Geometry check sheet. Reference: drawing and pictorial views, mm from the part's lowest x, y, z. A direction names the side the tool comes from. Coordinates: 2 decimals unless noted, no trailing zeros. Loops run counter-clockwise (first coordinate to the right, second up) from the corner with the lowest first, then second, coordinate; pieces in that order, holes last. Notation, with made-up numbers: M 62,-15.75 L 88,-15.75 A18 cw 88,-1.75 Z; hole C -14.75,61 d4. An arc over 180 degrees is marked long. Write item = value, one per line. Start each with the question number.
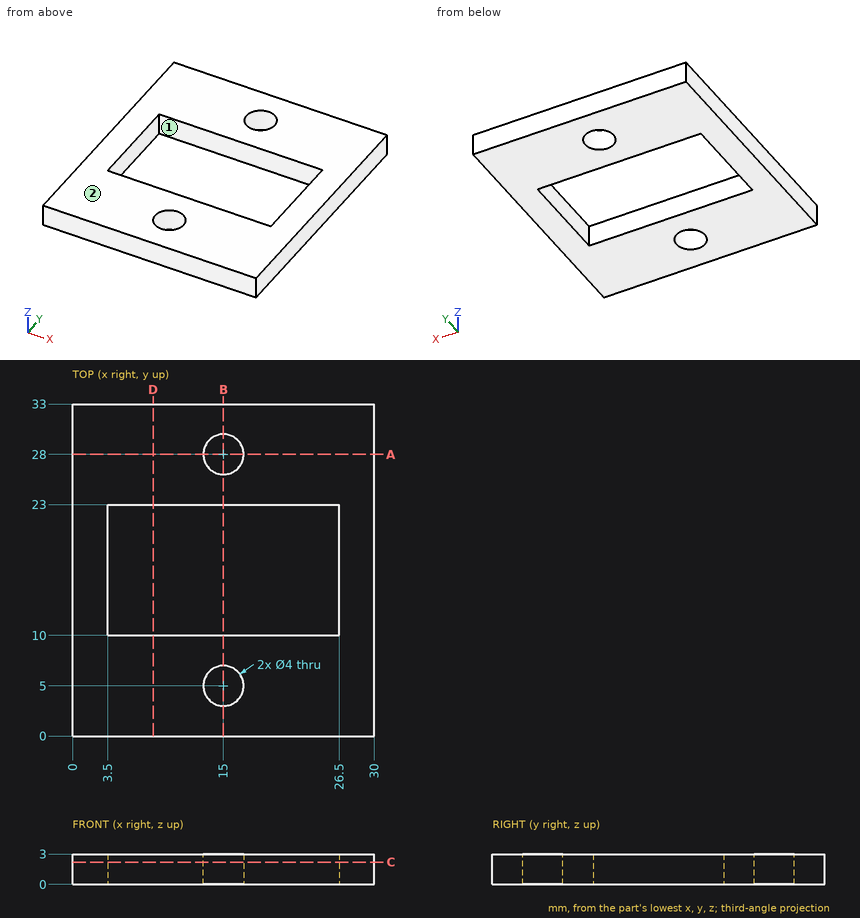
Q1. Scan lines: L1, parallel to Y at x = 15, z = 1.55; L2, parallel to Y at x = 5.75, z = 1.7; L3, parallel to X at y = 11, z = 0.5. Record each from-to range of solid material in increasing order. Write a range as [from, to].
Q2. Gauge pin test, flat end, axial feed: pin 1 (4.5 mm diameter, centred on x = 15, y = 28, fed in from +Z). Record the tip position at first contact, or that the pin passes through.
Q3. Sectioned sample at B-B on x = 15. Record the cut outline in (y, z), plus the area to 3 significant figures.
Q4. Sectioned sample at D-D on x = 8. Record the cut outline in (y, z).
Q5. Set-up check for the marked faces 1 and 2: record each of +Z, -Z, +X, -X, +Y, -Y from which the full face is reachable in a straight line by a thin tool's end or side.
Q6. Sectioned sample at A-A on y = 28. Record the cut outline in (x, z), plus the area to 3 significant figures.
Q7. Sectioned sample at C-C on z = 2.2. Record the cut outline in (x, y).
Solutions:
q1.L1 = [0, 3], [7, 10], [23, 26], [30, 33]
q1.L2 = [0, 10], [23, 33]
q1.L3 = [0, 3.5], [26.5, 30]
q2.pin_1 = 3
q3.outline = M 0,0 L 3,0 L 3,3 L 0,3 Z; M 7,0 L 10,0 L 10,3 L 7,3 Z; M 23,0 L 26,0 L 26,3 L 23,3 Z; M 30,0 L 33,0 L 33,3 L 30,3 Z
q3.area = 36.0 mm²
q4.outline = M 0,0 L 10,0 L 10,3 L 0,3 Z; M 23,0 L 33,0 L 33,3 L 23,3 Z
q5.face_1 = +Z, -Z
q5.face_2 = +Z, +X, -X, +Y, -Y
q6.outline = M 0,0 L 13,0 L 13,3 L 0,3 Z; M 17,0 L 30,0 L 30,3 L 17,3 Z
q6.area = 78.0 mm²
q7.outline = M 0,0 L 30,0 L 30,33 L 0,33 Z; hole M 3.5,10 L 26.5,10 L 26.5,23 L 3.5,23 Z; hole C 15,5 d4; hole C 15,28 d4
